from build123d import *

# Parameters (mm, degrees)
SKETCH1_W           = 15
SKETCH1_H           = 15
BOSS_EXTRUDE1_DEPTH = 10
SKETCH2_R           = 2.75
BOSS_EXTRUDE2_DEPTH = 3
SKETCH3_W           = 2.5
SKETCH3_H           = 5
BOSS_EXTRUDE3_DEPTH = 4
FILLET1_R           = 5
FILLET2_R           = 3
SKETCH4_W           = 5
SKETCH4_H           = 2
BOSS_EXTRUDE4_DEPTH = 1
FILLET3_R           = 1
SKETCH5_W           = 2.75
SKETCH5_H           = 7.677004104
CUT_EXTRUDE1_DEPTH  = 1
SKETCH6_R           = 1
CUT_EXTRUDE2_DEPTH  = 8
SKETCH7_R           = 0.875
BOSS_EXTRUDE5_DEPTH = 7.5
FILLET5_R           = 1


with BuildPart() as part:
    # Sketch1 → Boss-Extrude1 (new body)
    with BuildSketch(Plane.XY):
        Rectangle(SKETCH1_W, SKETCH1_H)
    extrude(amount=BOSS_EXTRUDE1_DEPTH)

    # Sketch2 → Boss-Extrude2 (add)
    with BuildSketch(Plane(origin=(0, 0, 0), x_dir=(-1, 0, 0), z_dir=(0, 0, -1))):
        Circle(SKETCH2_R)
    extrude(amount=BOSS_EXTRUDE2_DEPTH)

    # Sketch3 → Boss-Extrude3 (add)
    with BuildSketch(Plane(origin=(0, 7.5, 0), x_dir=(1, 0, 0), z_dir=(0, 1, 0))):
        Polygon((-2.5, 0), (0, 0), (2.5, 0), (2.5, 11.5), (-2.5, 11.5), align=None)
        with Locations((1.25, -2.5)):
            Rectangle(SKETCH3_W, SKETCH3_H)
        with Locations((-1.25, -2.5)):
            Rectangle(SKETCH3_W, SKETCH3_H)
    extrude(amount=BOSS_EXTRUDE3_DEPTH)

    # Fillet1
    # the kernel refuses this fillet: 5 mm, written as the material it adds along each edge
    with BuildSketch(Plane(origin=(2.5, 7.5, 5), x_dir=(0, 0, 1), z_dir=(-1, 0, 0))) as fillet1_piece_1:
        with BuildLine():
            CenterArc((4.898979486, 5), FILLET1_R, 191.536959033, 78.463040967)
            Line((0, 4), (-0.09797959, 3.98))
            ThreePointArc((-0.09797959, 3.98), (-0.1, 2), (-0.1, 0))
            Line((-0.1, 0), (0, -0.1))
            Line((0, -0.1), (4.898979486, -0.1))
            Line((4.898979486, -0.1), (4.898979486, 0))
        make_face()
    extrude(amount=5)

    # Fillet2
    fillet2_edges = [part.edges().sort_by_distance(p)[0] for p in [
        (0, 7.5, 0),
    ]]
    fillet(fillet2_edges, radius=FILLET2_R)

    # Sketch4 → Boss-Extrude4 (add)
    with BuildSketch(Plane.XZ.offset(-7.5)):
        with Locations((0, -10.5)):
            Rectangle(SKETCH4_W, SKETCH4_H)
    extrude(amount=BOSS_EXTRUDE4_DEPTH)

    # Fillet3
    fillet3_edges = [part.edges().sort_by_distance(p)[0] for p in [
        (0, 6.5, -11.5),
    ]]
    fillet(fillet3_edges, radius=FILLET3_R)

    # Sketch5 → Cut-Extrude1 (cut)
    with BuildSketch(Plane.XZ.offset(7.5)):
        with Locations((-1.375, 5)):
            Rectangle(SKETCH5_W, SKETCH5_H)
        with Locations((1.375, 5)):
            Rectangle(SKETCH5_W, SKETCH5_H)
    extrude(amount=-CUT_EXTRUDE1_DEPTH, mode=Mode.SUBTRACT)

    # Sketch6 → Cut-Extrude2 (cut)
    with BuildSketch(Plane(origin=(0, 0, 0), x_dir=(-1, 0, 0), z_dir=(0, 0, -1))):
        with Locations((-5, 0)):
            Circle(SKETCH6_R)
    extrude(amount=-CUT_EXTRUDE2_DEPTH, mode=Mode.SUBTRACT)

    # Sketch7 → Boss-Extrude5 (add)
    with BuildSketch(Plane(origin=(0, 0, 0), x_dir=(-1, 0, 0), z_dir=(0, 0, -1))):
        with Locations((5, 0)):
            Circle(SKETCH7_R)
    extrude(amount=BOSS_EXTRUDE5_DEPTH)

    # Fillet5
    fillet5_edges = [part.edges().sort_by_distance(p)[0] for p in [
        (0, -7.5, 0),
    ]]
    fillet(fillet5_edges, radius=FILLET5_R)


solid = part.part
Can you work these out from the model? Positions are in its coordinate system, mm. A direction names the side the tool comes from. Coordinates: 2 decimals unless noted, no trailing zeros. Order: outer loops, then holes, each group sorted by start corner. A loop starts at its lowest first (then second) coordinate and runs counter-clockwise, first axis right, second up. Notation, with made-up numbers: (-35.5, -32.75) - (20.5, -32.75) arc R14 ccw to (20.5, -14.75) - close; hole circle Ø4 at (69.25, -5.75). An arc over 180 degrees is marked (long way). Answer as a JSON object with one key per item and string values. Group by question number.
Q1. Imagine slicing it at C-C (x = 5). Please give me the cut outline in (y, z), and give its area (3 significant figures).
Q2. Will these pins go through, and if not, where does the flat tip stop? P1, Ø3, axis at x = 5, y = 0, coming from the -Z side; P2, Ø0.5, axis at x = 0, z = -10, coming from the -Y side; P3, Ø1.5, axis at x = 1, z = -6, coming from the -Y side; P4, Ø4.5, axis at x = 1, z = 6, coming from the -Y side.
Q3. Imagine slicing it at D-D (z = -8.5). Please give me the cut outline in (x, y), and give its area (3 significant figures).
Q4. I need wall thicknesses on line 1 (Y direction, x = 5, z = 2.75); line 2 (Z direction, x = 3.75, y = 3.25); line 3 (Y direction, x = -0.5, z = -8.75). Which ranges of each line are inside material? Lowest first, please. Write a range as from..to.
Q5. On a 3-axis mill with a long thin cutter (end or side, diameter ignored), from which of +Z, -Z, +X, -X, +Y, -Y can I reach the whole of each face in a straight line? I mean faces 1 (the face through (0.596, -2.685, -1.479)), 2 (the face through (0, 10, -11.5)), 3 (the face through (0, 0, -3)), 4 (the face through (0, -6.5, 5)). Say none if no direction works.
Q6. Imagine slicing it at A-A (y = 0). Please give me the cut outline in (x, z) (3 decimals).
Q7. We'd pull the mould along Z, two halves only. Please class faces 5 (the face through (0, 7, -9.5)), 6 (the face through (7.5, 0, 5)), 7 (the face through (-5, 0, -7.5)): +Z half, -Z half, draft (parallel to the pull), parting line (faces both ways), or undercut.
Q8. Imagine slicing it at B-B (z = -4.25). Please give me the cut outline in (x, y) (3 decimals), and give its area (3 significant figures).
Determined:
{
 "1": {"outline": "(-7.5, 1) arc R1 ccw to (-6.5, 0) - (-1, 0) - (-1, 8) - (1, 8) - (1, 0) - (7.5, 0) - (7.5, 10) - (-7.5, 10) - close", "area": "134 mm2"},
 "2": {"P1": "stops at z = 0", "P2": "stops at y = 6.5", "P3": "stops at y = 7.5", "P4": "stops at y = -7.5"},
 "3": {"outline": "(-2.5, 7.5) - (2.5, 7.5) - (2.5, 11.5) - (-2.5, 11.5) - close", "area": "20.0 mm2"},
 "4": {"line 1": "y = -7.5..-1, 1..7.5", "line 2": "z = 0..10", "line 3": "y = 7.5..11.5"},
 "5": {"face 1": "-Z", "face 2": "-Z, +X, -X, +Y, -Y", "face 3": "-Z, +X, -Y", "face 4": "-Y"},
 "6": {"outline": "(-7.5, 0) - (-5.875, 0) - (-5.875, -7.5) - (-4.125, -7.5) - (-4.125, 0) - (-2.75, 0) - (-2.75, -3) - (2.75, -3) - (2.75, 0) - (4, 0) - (4, 8) - (6, 8) - (6, 0) - (7.5, 0) - (7.5, 10) - (-7.5, 10) - close"},
 "7": {"face 5": "undercut", "face 6": "draft", "face 7": "-Z half"},
 "8": {"outline": "circle Ø1.75 at (-5, 0); (-2.5, 7.5) - (2.5, 7.5) - (2.5, 11.5) - (-2.5, 11.5) - close", "area": "22.4 mm2"}
}
